from build123d import *

# Parameters (mm, degrees)
SKETCH1_R                                         = 10.414
BOSS_EXTRUDE1_DEPTH                               = 3.81
SKETCH2_R                                         = 5.715
CUT_EXTRUDE1_DEPTH                                = 16.212458447
SKETCH3_R                                         = 6.35
CUT_EXTRUDE3_DEPTH                                = 1.27
CSK_FOR_0_FLAT_HEAD_MACHINE_SCREW_100_D           = 1.6129
CSK_FOR_0_FLAT_HEAD_MACHINE_SCREW_100_CSINK_D     = 3.0226
CSK_FOR_0_FLAT_HEAD_MACHINE_SCREW_100_CSINK_ANGLE = 100
CIRPATTERN1_COUNT                                 = 3


with BuildPart() as part:
    # Sketch1 → Boss-Extrude1 (new body)
    with BuildSketch(Plane.XY):
        with Locations(Location((0, 0, 0), (0, 0, 180))):
            Circle(SKETCH1_R)
    extrude(amount=BOSS_EXTRUDE1_DEPTH)

    # Sketch2 → Cut-Extrude1 (cut, through all)
    with BuildSketch(Plane.XY.offset(3.81)):
        Circle(SKETCH2_R)
    extrude(amount=-CUT_EXTRUDE1_DEPTH, mode=Mode.SUBTRACT)

    # Sketch3 → Cut-Extrude3 (cut)
    with BuildSketch(Plane(origin=(0, 0, 0), x_dir=(-1, 0, 0), z_dir=(0, 0, -1))):
        Circle(SKETCH3_R)
    extrude(amount=-CUT_EXTRUDE3_DEPTH, mode=Mode.SUBTRACT)

    # CSK for #0 Flat Head Machine Screw (100)1 (through all)
    with Locations(Plane.XY.offset(3.81)):
        with Locations((-5.104644358, -6.648347913)):
            csk_for_0_flat_head_machine_screw_100 = CounterSinkHole(CSK_FOR_0_FLAT_HEAD_MACHINE_SCREW_100_D / 2, CSK_FOR_0_FLAT_HEAD_MACHINE_SCREW_100_CSINK_D / 2, counter_sink_angle=CSK_FOR_0_FLAT_HEAD_MACHINE_SCREW_100_CSINK_ANGLE)

    # CirPattern1: CSK for #0 Flat Head Machine Screw (100)1 ×3 about axis
    cirpattern1_axis = Axis((0, 0, 0), (0, 0, 1))
    for i in range(1, CIRPATTERN1_COUNT):
        add(csk_for_0_flat_head_machine_screw_100.rotate(cirpattern1_axis, i * 360 / CIRPATTERN1_COUNT), mode=Mode.SUBTRACT)


solid = part.part
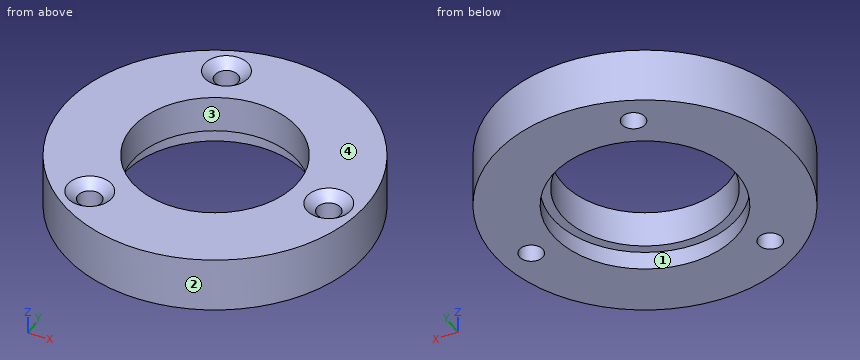
Work out the finished part from the listing and answer in its coordinate system (mm). Face numbers are marked on the shaded views. Give positions to 0.01 mm unless a question says otherwise; leave off trailing zeros. Write each loop counter-clockwise with the first axis right and the second up, starting at its lowest first coordinate (ties: lowest second). Pieces come first, ordered by that corner, then holes. Notation, with made-up numbers: (-16, 5) - (1, 5) arc R24 ccw to (1, 44) - close; hole circle Ø6 at (-21.5, 24). An arc over 180 degrees is marked (long way). One line per item, written item: value. Start each with the question number.
1. For a pull along Y with two mould halves and no side action, classify the marked faces 1, 2, 3 and 4 as +Y half, -Y half, draft (parallel to the pull), parting line (faces both ways), or undercut.
2. Find section C-C (z = 2.4). Write down the section's boundary in (x, y) (3 decimals), then the cut area to 3 significant figures.
3. Given pin 1 (9 mm diameter, centred on x = 0, y = 0, fed in from -Z), flat-ended and moving along its own axis, determine where the tip first touches the part or whether it passes through.
4. Consider probe 1 along Y at (x, z) = (0, 0.35); probe 2 along Y at (x, z) = (8.25, 2.15); probe 3 along Y at (x, z) = (-4.5, 1.05). Determine where each line is inside the solid, lowest interval first.
5. Find section D-D (z = 0.45). Write down the section's boundary in (x, y), then the cut area to 3 significant figures.
6. Find section B-B (x = 0). Write down the section's boundary in (y, z) (3 decimals).
7. Find section A-A (y = -4). Write down the section's boundary in (x, z).
Geometry results:
1. face 1: undercut
1. face 2: parting line
1. face 3: undercut
1. face 4: draft
2. outline: circle Ø20.828 at (0, 0); hole circle Ø1.613 at (-5.105, -6.648); hole circle Ø11.43 at (0, 0); hole circle Ø1.613 at (-3.205, 7.745); hole circle Ø1.613 at (8.31, -1.097)
2. area: 232 mm2
3. pin 1: through
4. probe 1: -10.41 to -6.35, 6.35 to 10.41
4. probe 2: -6.36 to -1.9, -0.29 to 6.36
4. probe 3: -9.39 to -7.18, -6.11 to -4.48, 4.48 to 9.39
5. outline: circle Ø20.83 at (0, 0); hole circle Ø12.7 at (0, 0); hole circle Ø1.61 at (-5.1, -6.65); hole circle Ø1.61 at (-3.21, 7.74); hole circle Ø1.61 at (8.31, -1.1)
5. area: 208 mm2
6. outline: (-10.414, 0) - (-6.35, 0) - (-6.35, 1.27) - (-5.715, 1.27) - (-5.715, 3.81) - (-10.414, 3.81) - close; (5.715, 1.27) - (6.35, 1.27) - (6.35, 0) - (10.414, 0) - (10.414, 3.81) - (5.715, 3.81) - close
7. outline: (-9.62, 0) - (-4.93, 0) - (-4.93, 1.27) - (-4.08, 1.27) - (-4.08, 3.81) - (-9.62, 3.81) - close; (4.08, 1.27) - (4.93, 1.27) - (4.93, 0) - (9.62, 0) - (9.62, 3.81) - (4.08, 3.81) - close
